```python
from build123d import *

# Parameters (mm, degrees)
F0_R      = 19.25
F1_DEPTH  = 1
F2_R      = 19.25
F3_DEPTH  = 65
F7_DEPTH  = 25
F10_DEPTH = 8
F14_DEPTH = 25
F16_DEPTH = 25
F17_R     = 2
F18_R     = 15
F19_W     = 3
F19_H     = 20
F20_DEPTH = 50
F21_R     = 1
F4_R      = 16.5
F22_DEPTH = 58
F23_R     = 10


with BuildPart() as f1:
    # F0 (on Right) → F1 (new body)
    with BuildSketch(Plane.YZ):
        Circle(F0_R)
    extrude(amount=F1_DEPTH)

    # F2 (on face) → F3 (join)
    with BuildSketch(Plane(origin=(0, 0, 0), x_dir=(0, -1, 0), z_dir=(-1, 0, 0))):
        Circle(F2_R)
    extrude(amount=F3_DEPTH)

    # F6 (on offset) → F7 (cut)
    with BuildSketch(Plane.XY.offset(20)):
        Polygon((-59.3079618843, 7.4748665604), (-65, 7.4748665604), (-65, 3.8748665604), (-59.3079618843, 3.8748665604), (-57.9855095289, -3.6251334396), (-54.4402016181, -3), (-56.287203212, 7.4748665604), align=None)
    extrude(amount=-F7_DEPTH, mode=Mode.SUBTRACT)

    # F9 (on offset) → F10 (cut)
    with BuildSketch(Plane.XY.offset(-20)):
        Polygon((-65, -3.8748665604), (-65, -7.4748665604), (-59.3081739576, -7.4748665604), (-56.2874152853, -7.4748665604), (-54.4404136914, 3), (-57.9857216023, 3.6251334396), (-59.3081739576, -3.8748665604), align=None)
    extrude(amount=F10_DEPTH, mode=Mode.SUBTRACT)

    # F13 (on offset) → F14 (cut)
    with BuildSketch(Plane.XZ.offset(-20)):
        Polygon((-65, -3.8748665604), (-65, -7.4748665604), (-59.3079618843, -7.4748665604), (-56.287203212, -7.4748665604), (-54.4402016181, 3), (-57.9855095289, 3.6251334396), (-59.3079618843, -3.8748665604), align=None)
    extrude(amount=F14_DEPTH, mode=Mode.SUBTRACT)

    # F15 (on offset) → F16 (cut)
    with BuildSketch(Plane.XZ.offset(20)):
        Polygon((-59.3079618843, 7.4748665604), (-65, 7.4748665604), (-65, 3.8748665604), (-59.3079618843, 3.8748665604), (-57.9855095289, -3.6251334396), (-54.4402016181, -3), (-56.287203212, 7.4748665604), align=None)
    extrude(amount=-F16_DEPTH, mode=Mode.SUBTRACT)

    # F17
    f17_edges = [f1.edges().sort_by_distance(p)[0] for p in [
        (-59.308174, -3.874867, -15.427989),
        (-59.307962, 13.165422, -3.874867),
        (-59.307962, -0.562567, -3.874867),
        (-59.307962, 3.874867, 13.165422),
        (-59.307962, 3.874867, 0),
        (-59.307962, -7.490556, 3.874867),
    ]]
    fillet(f17_edges, radius=F17_R)

    # F18
    f18_edges = [f1.edges().sort_by_distance(p)[0] for p in [
        (1, -19.25, 0),
    ]]
    fillet(f18_edges, radius=F18_R)

    # F19 (on offset) → F20 (cut)
    with BuildSketch(Plane.XZ.offset(-20)):
        with Locations((-19.5, 0)):
            Rectangle(F19_W, F19_H)
        with Locations((-25.5, 0)):
            Rectangle(F19_W, F19_H)
        with Locations((-31.5, 0)):
            Rectangle(F19_W, F19_H)
        with Locations((-37.5, 0)):
            Rectangle(F19_W, F19_H)
    extrude(amount=F20_DEPTH, mode=Mode.SUBTRACT)

    # F21
    f21_edges = [f1.edges().sort_by_distance(p)[0] for p in [
        (-65, 17.033005, 8.968793),
        (-65, 8.968793, -17.033005),
        (-65, -19.151241, 1.947424),
        (-65, -8.968793, 17.033005),
        (-65, -7.474867, -14.869736),
        (-65, -3.874867, -15.427989),
        (-65, -0.562567, -3.874867),
        (-65, 13.165422, -3.874867),
        (-65, 6.369736, -7.474867),
        (-65, 7.474867, 6.932303),
        (-65, 3.874867, 0),
        (-65, 3.874867, 13.165422),
        (-65, -7.490556, 3.874867),
        (-65, -6.932303, 7.474867),
        (-65, -16.038293, -10.645922),
    ]]
    fillet(f21_edges, radius=F21_R)

    # F4 (on face) → F22 (cut)
    with BuildSketch(Plane(origin=(-65, 0, 0), x_dir=(0, -1, 0), z_dir=(-1, 0, 0))):
        Circle(F4_R)
    extrude(amount=-F22_DEPTH, mode=Mode.SUBTRACT)

    # F23
    f23_edges = [f1.edges().sort_by_distance(p)[0] for p in [
        (-7, 16.5, 0),
    ]]
    fillet(f23_edges, radius=F23_R)


solid = f1.part
```
The model under review builds one solid part; all positions refer to its coordinate system, in mm. A direction names the side the tool comes from. Coordinates: 2 decimals unless noted, no trailing zeros. Order: outer loops, then holes, each group sorted by start corner. A loop starts at its lowest first (then second) coordinate and runs counter-clockwise, first axis right, second up. Notation, with made-up numbers: (53, 12) -> (76, 12) arc R11 cw to (76, 30) -> close; hole circle Ø5 at (79.5, 58). An arc over 180 degrees is marked (long way). Answer in a Markdown table with one row per item. Add a question column.
Item 1: We need section A-A on x = -51. Write out the cut boundary in (y, z), plus the area to 3 significant figures.
Item 2: To check wall thickness, follow probe 1 along Y at (x, z) = (-35, 0); probe 2 along Z at (x, y) = (-43, 7.5). State the ranges of each line that lie inside material, in increasing order.
Item 3: Clearance check with flat-ended pins moving along their axes: pin 1 (5 mm diameter, centred on x = -10.5, z = -8, fed in from -Y); pin 2 (3.5 mm diameter, centred on x = -19, y = 15, fed in from -Z); pin 3 (5 mm diameter, centred on y = 17, z = -4, fed in from +X). State where each tip first meets the part, or that it passes through.
Item 4: Mouldability with a two-part tool opening along Z and no side actions: class faces 6 (the cylindrical face through (-59.686, -3.394, -17.558)), 7 (the flat face through (-39, -17, 0)) as +Z half, -Z half, draft (parallel to the pull), parting line (faces both ways), or undercut.
Item 5: Machinability: for faces 1 (the flat face through (-60, -7.475, -16)), 2 (the flat face through (-56.19, 3.31, -17.58)), 3 (the flat face through (-38, 15, 10)), 4 (the flat face through (-55.377, 17.516, -2.311)), 5 (the flat face through (-56.238, -17.576, -3.317)), which of the approach directions +Z, -Z, +X, -X, +Y, -Y give a long, thin tool a straight path to every point of the face, cutting with its end or side? Answer none if there is none.
Item 6: We need section B-B on y = 0. Give the number of separate pieces and of enclosed holes in the cut face, plus the area to 3 significant figures.
Final values:
| question | item | result |
|---|---|---|
| 1 | outline | circle Ø38.5 at (0, 0); hole circle Ø33 at (0, 0) |
| 1 | area | 309 mm2 |
| 2 | probe 1 | y = -19.25 to -16.5, 16.5 to 19.25 |
| 2 | probe 2 | z = -17.73 to -14.7, 14.7 to 17.73 |
| 3 | pin 1 | stops at y = -18.17 |
| 3 | pin 2 | stops at z = -13.96 |
| 3 | pin 3 | stops at x = -3.5 |
| 4 | face 6 | draft |
| 4 | face 7 | undercut |
| 5 | face 1 | -Z, -X |
| 5 | face 2 | -Z |
| 5 | face 3 | +Y, -Y |
| 5 | face 4 | +Y |
| 5 | face 5 | -Y |
| 6 | separate pieces | 3 |
| 6 | enclosed holes | 0 |
| 6 | area | 553 mm2 |
